Build history of the part. All positions in model axes, mm. A direction names the side the tool comes from. Round coordinates to 2 decimals unless told otherwise and drop trailing zeros. Order: outer loops, then holes, each group sorted by start corner. A loop starts at its lowest first (then second) coordinate and runs counter-clockwise, first axis right, second up. Notation, with made-up numbers: M -6,61 L 32,61 A15 ccw 32,77 Z; hole C -26.75,-37 d10. An arc over 180 degrees is marked long. One line per question, with ' | ' between items. Start each with the question number.
from build123d import *

# Parameters (mm, degrees)
F0_W     = 234.95
F0_H     = 25.4
F1_DEPTH = 12.7
F2_W     = 6.35
F2_H     = 6.35
F3_DEPTH = 234.951
F5_DEPTH = 25.401
F6_W     = 6.35
F6_H     = 6.35
F7_DEPTH = 166.135738
F8_W     = 6.35
F8_H     = 6.35
F9_DEPTH = 166.135738


with BuildPart() as f1:
    # F0 (on Right) → F1 (new body)
    with BuildSketch(Plane.YZ):
        with Locations((0, 12.7)):
            Rectangle(F0_W, F0_H)
    extrude(amount=F1_DEPTH)

    # F2 (on face) → F3 (cut, through all)
    with BuildSketch(Plane(origin=(0, 117.475, 0), x_dir=(-1, 0, 0), z_dir=(0, 1, 0))):
        with Locations((-3.175, 15.875)):
            Rectangle(F2_W, F2_H)
    extrude(amount=-F3_DEPTH, mode=Mode.SUBTRACT)

    # F4 (on face) → F5 (cut, through all)
    with BuildSketch(Plane.XY.offset(25.4)):
        Polygon((0, 117.475), (0, 104.775), (12.7, 117.475), align=None)
        Polygon((12.7, -117.475), (0, -104.775), (0, -117.475), align=None)
    extrude(amount=-F5_DEPTH, mode=Mode.SUBTRACT)

    # F6 (on face) → F7 (cut, through all)
    with BuildSketch(Plane(origin=(-52.3875, -52.3875, 0), x_dir=(0.707107, -0.707107, 0), z_dir=(-0.707107, -0.707107, 0))):
        with Locations((88.872625, 12.7)):
            Rectangle(F6_W, F6_H)
    extrude(amount=-F7_DEPTH, mode=Mode.SUBTRACT)

    # F8 (on face) → F9 (cut, through all)
    with BuildSketch(Plane(origin=(-52.3875, 52.3875, 0), x_dir=(-0.707107, -0.707107, 0), z_dir=(-0.707107, 0.707107, 0))):
        with Locations((-88.872625, 12.7)):
            Rectangle(F8_W, F8_H)
    extrude(amount=-F9_DEPTH, mode=Mode.SUBTRACT)


solid = f1.part
Item 1: Wall check: line 1 along Z through (x, y) = (5.25, -89.5); line 2 along Y through (x, z) = (3.75, 4) (3 decimals); line 3 along Y through (x, z) = (8.25, 11). Give the ranges that are in metal, low to high. Write a range as [from, to].
Item 2: Tool access for faces 1 (the face through (12.7, -2, 13)), 2 (the face through (3, 2, 19.05)), 3 (the face through (10.424, 110.771, 12.656)), 4 (the face through (0, -1, 22)), 5 (the face through (12, -113, 9.525)): list every direction of +Z, -Z, +X, -X, +Y, -Y with a clear straight run to the whole face (end or side of a thin tool).
Item 3: Flat gauge pins, fed straight in: pin 1 (6 mm diameter, centred on x = 9, z = 17.5, fed in from -Y) (3 decimals); pin 2 (3 mm diameter, centred on y = -50.5, z = 16.5, fed in from -X). Where does each tip first touch, or does it go through?
Item 4: Cut at B-B on x = 4. Write the cut outline in (y, z) (3 decimals).
Item 5: Cut at C-C on z = 22.75. Write the cut outline in (x, y) (3 decimals).
Item 6: Cut at A-A on y = -102. Write the cut outline in (x, z), then the cut area to 3 significant figures.
Item 7: Two-plate mould, pull along Z, no slides. Class faces 6 (the face through (6, -2, 25.4)), 7 (the face through (10.424, -110.771, 12.656)), 8 (the face through (7.672, 112.447, 12.878)): +Z half, -Z half, draft (parallel to the pull), parting line (faces both ways), or undercut.
Results found:
1) line 1: z = [0, 12.7], [19.05, 25.4] | line 2: y = [-108.525, 108.525] | line 3: y = [-112.94, 112.94]
2) face 1: +Z, -Z, +X, +Y, -Y | face 2: -X, +Y, -Y | face 3: +X, +Y | face 4: +Z, -Z, -X, +Y, -Y | face 5: +X, -Y
3) pin 1: stops at y = -116.775 | pin 2: stops at x = 6.35
4) outline: M -108.775,0 L 108.775,0 L 108.775,12.7 L -108.775,12.7 Z; M -108.775,19.05 L 108.775,19.05 L 108.775,25.4 L -108.775,25.4 Z
5) outline: M 0,-104.775 L 12.7,-117.475 L 12.7,117.475 L 0,104.775 Z
6) outline: M 0,0 L 12.7,0 L 12.7,25.4 L 0,25.4 L 0,19.05 L 6.35,19.05 L 6.35,12.7 L 0,12.7 Z | area: 282 mm^2
7) face 6: +Z half | face 7: undercut | face 8: draft
